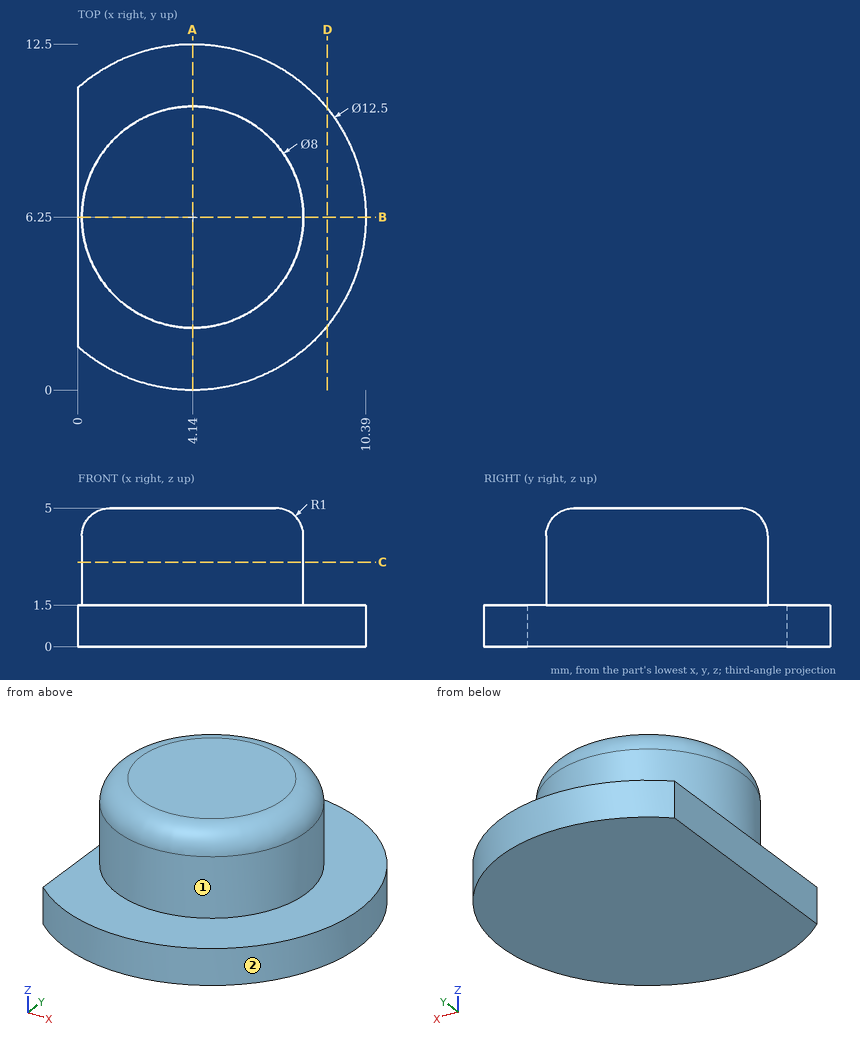
Geometry check sheet. Reference: drawing and pictorial views, mm from the part's lowest x, y, z. A direction names the side the tool comes from. Give positions to 0.01 mm unless a question says otherwise; leave off trailing zeros. Order: outer loops, then holes, each group sorted by start corner. A loop starts at its lowest first (then second) coordinate and runs counter-clockwise, first axis right, second up. Notation, with made-up numbers: M -20,8 L -7,8 A5 cw -7,14 Z; hole C 66,76 d11. An arc over 180 degrees is marked long. Use one line per item in the form item = value. Start each with the question number.
Q1. Scan lines: line 1 along Z through (x, y) = (9, 8.25); line 2 along Y through (x, z) = (2.25, 0.75); line 3 along X through (y, z) = (10, 0.55). Record each from-to range of solid material in increasing order. Write a range as [from, to].
Q2. Section check C-C (z = 3.05). Enter the section's corners in (x, y).
Q3. Section check B-B (y = 6.25). Enter the section's corners in (x, z).
Q4. Section check A-A (x = 4.14). Enter the section's corners in (y, z), then the cut area to 3 significant figures.
Q5. Go/stop test with a flat-tipped pin: pin 1 Ø3 at (x, y) = (3.5, 1.5) entering from +Z. Record where the tip stops, or that it passes through.
Q6. Section check D-D (x = 9). Enter the section's corners in (y, z).
Q7. Access from +Z, -Z, +X, -X, +Y, -Y to the whole of each face (thin tool, end or side, straight path). Record for the marked faces 1 and 2.
Evaluation:
q1.line_1 = [0, 1.5]
q1.line_2 = [0.29, 12.21]
q1.line_3 = [0, 9.14]
q2.outline = C 4.14,6.25 d8
q3.outline = M 0,0 L 10.39,0 L 10.39,1.5 L 8.14,1.5 L 8.14,4 A1 ccw 7.14,5 L 1.14,5 A1 ccw 0.14,4 L 0.14,1.5 L 0,1.5 Z
q4.outline = M 0,0 L 12.5,0 L 12.5,1.5 L 10.25,1.5 L 10.25,4 A1 ccw 9.25,5 L 3.25,5 A1 ccw 2.25,4 L 2.25,1.5 L 0,1.5 Z
q4.area = 46.3 mm2
q5.pin_1 = 4.96
q6.outline = M 2.32,0 L 10.18,0 L 10.18,1.5 L 2.32,1.5 Z
q7.face_1 = +Z
q7.face_2 = +Z, -Z
